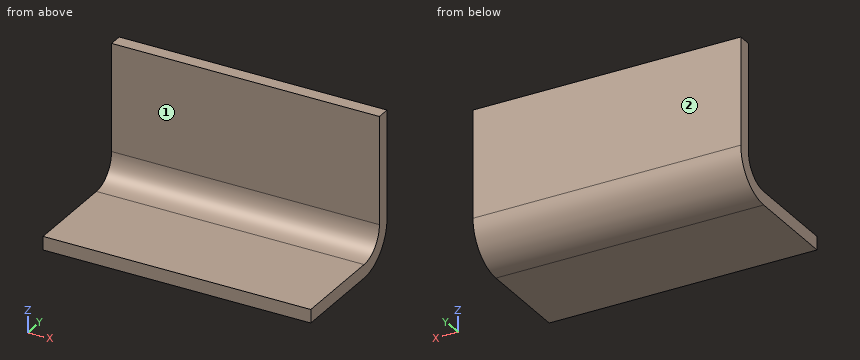
```python
from build123d import *

# Parameters (mm, degrees)
SKETCH_1_W                 = 20
SKETCH_1_H                 = 10
BASEPLATE_DEPTH            = 1
EDGEFLANGE_STRIP_W         = 8
EDGEFLANGE_STRIP_H         = 1
EDGEFLANGE_STRIP_CUT_DEPTH = 20
EDGEFLANGE_DEPTH           = 20
EDGEFLANGE_FLAT_DEPTH      = 1


# Sheet-metal steps are written as plain solids
with BuildPart() as part:
    # Sketch 1 → BasePlate (new body)
    with BuildSketch(Plane.XY):
        with Locations((10, 5)):
            Rectangle(SKETCH_1_W, SKETCH_1_H)
    extrude(amount=-BASEPLATE_DEPTH)

    # EdgeFlange strip (across the edge) → EdgeFlange strip cut (cut)
    with BuildSketch(Plane(origin=(20, 10, 0), x_dir=(0, -1, 0), z_dir=(-1, 0, 0))):
        with Locations((-1, -0.5)):
            Rectangle(EDGEFLANGE_STRIP_W, EDGEFLANGE_STRIP_H)
    extrude(amount=EDGEFLANGE_STRIP_CUT_DEPTH, mode=Mode.SUBTRACT)

    # EdgeFlange bend section (across the edge) → EdgeFlange (add)
    with BuildSketch(Plane(origin=(20, 10, 0), x_dir=(0, -1, 0), z_dir=(-1, 0, 0))):
        with BuildLine():
            Line((0, 2), (1, 2))
            ThreePointArc((1, 2), (1.585786438, 0.585786438), (3, 0))
            Line((3, 0), (3, -1))
            ThreePointArc((3, -1), (0.878679656, -0.121320344), (0, 2))
        make_face()
    extrude(amount=EDGEFLANGE_DEPTH)

    # EdgeFlange profile (on flange) → EdgeFlange flat (add)
    with BuildSketch(Plane(origin=(0, 10, 0), x_dir=(-1, 0, 0), z_dir=(0, 1, 0))):
        Polygon((-20, 10), (-20, 2), (0, 2), (0, 10), (-2, 10), (-18, 10), align=None)
    extrude(amount=-EDGEFLANGE_FLAT_DEPTH)


solid = part.part
```
The model under review builds one solid part; all positions refer to its coordinate system, in mm. Face numbers are marked on the shaded views. A direction names the side the tool comes from. Round coordinates to 2 decimals unless told otherwise and drop trailing zeros. Write each loop counter-clockwise with the first axis right and the second up, starting at its lowest first coordinate (ties: lowest second). Pieces come first, ordered by that corner, then holes.
(1) We need section A-A on x = 5.75. Give the boundary of the cut face in (y, z).
(2) Wall thickness on L1, parallel to Z at x = 11.75, y = 1; L2, parallel to Y at x = 3.75, z = 3; L3, parallel to Z at x = 13.25, y = 9.25: over which ranges is each line inside the solid? List them lowest first.
(3) We need section C-C on z = 1. Give the boundary of the cut face in (x, y), and give its area (3 significant figures).
(4) Machinability: for the marked faces 1 and 2, which of the approach directions +Z, -Z, +X, -X, +Y, -Y give a long, thin tool a straight path to every point of the face, cutting with its end or side? Answer none if there is none.
(5) We need section B-B on y = 2.5. Give the boundary of the cut face in (x, z), and give its area (3 significant figures).
(6) Insertion check: pin 1 (4 mm diameter, centred on x = 7.5, z = 6.5, fed in from -Y). The pin has a flat end and moves straight along its axis. Give the tip position at first contact, or say it passes through.
Findings below:
1. outline: (0, -1) - (7, -1) arc R3 ccw to (10, 2) - (10, 10) - (9, 10) - (9, 2) arc R2 cw to (7, 0) - (0, 0) - close
2. L1: z = -1 to 0
2. L2: y = 9 to 10
2. L3: z = 0.02 to 10
3. outline: (0, 8.73) - (20, 8.73) - (20, 9.83) - (0, 9.83) - close
3. area: 21.9 mm2
4. face 1: +Z, +X, -X, -Y
4. face 2: +Z, -Z, +X, -X, +Y
5. outline: (0, -1) - (20, -1) - (20, 0) - (0, 0) - close
5. area: 20.0 mm2
6. pin 1: stops at y = 9
